```python
from build123d import *

# Parameters (mm, degrees)
F0_W     = 45
F0_H     = 45
F3_DEPTH = 3
F4_R     = 5
F1_W     = 25
F1_H     = 25
F5_DEPTH = 3
F6_R     = 5
F2_W     = 25
F2_H     = 25
F7_DEPTH = 3
F8_R     = 5
F10_D    = 3
F12_D    = 3


with BuildPart() as f3:
    # F0 (on Top) → F3 (new body)
    with BuildSketch(Plane.XY):
        with Locations((-22.5, -22.5)):
            Rectangle(F0_W, F0_H)
    extrude(amount=F3_DEPTH)

    # F4
    f4_edges = [f3.edges().sort_by_distance(p)[0] for p in [
        (-45, -45, 1.5),
    ]]
    fillet(f4_edges, radius=F4_R)

    # F1 (on Right) → F5 (join)
    with BuildSketch(Plane.YZ):
        with Locations((-12.5, 12.5)):
            Rectangle(F1_W, F1_H)
    extrude(amount=-F5_DEPTH)

    # F6
    f6_edges = [f3.edges().sort_by_distance(p)[0] for p in [
        (-1.5, -25, 25),
    ]]
    fillet(f6_edges, radius=F6_R)

    # F2 (on Front) → F7 (join)
    with BuildSketch(Plane.XZ):
        with Locations((-12.5, 12.5)):
            Rectangle(F2_W, F2_H)
    extrude(amount=F7_DEPTH)

    # F8
    f8_edges = [f3.edges().sort_by_distance(p)[0] for p in [
        (-25, -1.5, 25),
    ]]
    fillet(f8_edges, radius=F8_R)

    # F10 (through all)
    with Locations(Plane.XZ.offset(3)):
        with Locations((-16, 16)):
            Hole(F10_D / 2)

    # F12 (through all)
    with Locations(Plane(origin=(-3, 0, 0), x_dir=(0, -1, 0), z_dir=(-1, 0, 0))):
        with Locations((16, 16)):
            Hole(F12_D / 2)


solid = f3.part
```
The listing builds one solid part. Answer for the finished solid, in the listing's coordinates (mm). A direction names the side the tool comes from. Give positions to 0.01 mm unless a question says otherwise; leave off trailing zeros. Write each loop counter-clockwise with the first axis right and the second up, starting at its lowest first coordinate (ties: lowest second). Pieces come first, ordered by that corner, then holes. Notation, with made-up numbers: (64, -17) - (105, -17) arc R20 cw to (105, -3) - close; hole circle Ø7 at (-17.75, 70.5). An arc over 180 degrees is marked (long way). Use one line per item in the form item = value. Start each with the question number.
1) Flat-ended cylindrical pins translate along their axes: pin 1 Ø11 at (y, z) = (-13, 10) entering from -X; pin 2 Ø4 at (x, z) = (-20.5, 6) entering from +Y; pin 3 Ø0.9 at (x, z) = (-1.5, 15.5) entering from -Y; pin 4 Ø2 at (x, z) = (-16.5, 9) entering from -Y. Find the tip coordinate at first contact, or state that the pin passes through.
2) The mould has two halves that part along Z. Classify faces 1 (the face through (-23, -22, 0)), 2 (the face through (-2, -23, 24)), 3 (the face through (-14.5, -1.48, 16.07)), 4 (the face through (-14, -3, 14)): pulls with the +Z half, pulls with the -Z half, needs draft (parallel to the pull), parting line crosses it, or undercut.
3) Consider line 1 along Z through (x, y) = (-16, -1.95); line 2 along Y through (x, z) = (-13.5, 9); line 3 along Z through (x, y) = (-12, -9.5). Determine where each line is inside the solid, lowest interval first. Write a range as from..to.
4) Find section D-D on x = -4. Determine the outline of the cut face in (y, z), plus the area to 3 significant figures.
5) Find section A-A on x = -16. Determine the outline of the cut face in (y, z), plus the area to 3 significant figures.
6) A tool of negligible diameter and unlimited length cuts with its end or side. For faces 5 (the face through (0, -13, 12)), 6 (the face through (-25, -1, 11)), 7 (the face through (-3, -14, 14)), 8 (the face through (-2.5, -5.6, 25)), 9 (the face through (-1, -25, 11)), from which of +Z, -Z, +X, -X, +Y, -Y can it reach the whole face along a straight path? Write none if from no direction.
7) Find section B-B on z = 16. Determine the outline of the cut face in (x, y).
Geometry results:
q1.pin_1 = -3
q1.pin_2 = 0
q1.pin_3 = -25
q1.pin_4 = -3
q2.face_1 = pulls with the -Z half
q2.face_2 = pulls with the +Z half
q2.face_3 = undercut
q2.face_4 = needs draft
q3.line_1 = 0..14.5, 17.5..25
q3.line_2 = -3..0
q3.line_3 = 0..3
q4.outline = (-45, 0) - (0, 0) - (0, 25) - (-3, 25) - (-3, 3) - (-45, 3) - close
q4.area = 201 mm2
q5.outline = (-45, 0) - (0, 0) - (0, 14.5) - (-3, 14.5) - (-3, 3) - (-45, 3) - close; (-3, 17.5) - (0, 17.5) - (0, 25) - (-3, 25) - close
q5.area = 192 mm2
q6.face_5 = +Z, -Z, +X, +Y, -Y
q6.face_6 = +Z, -X, +Y, -Y
q6.face_7 = +Z, -X, -Y
q6.face_8 = +Z, +X, -X, +Y, -Y
q6.face_9 = +Z, +X, -X, -Y
q7.outline = (-25, -3) - (-17.5, -3) - (-17.5, 0) - (-25, 0) - close; (-14.5, -3) - (-3, -3) - (-3, -14.5) - (0, -14.5) - (0, 0) - (-14.5, 0) - close; (-3, -25) - (0, -25) - (0, -17.5) - (-3, -17.5) - close
